Geometry check sheet. Reference: drawing and pictorial views, mm from the part's lowest x, y, z. Give positions to 0.01 mm unless a question says otherwise; leave off trailing zeros. Order: outer loops, then holes, each group sorted by start corner. A loop starts at its lowest first (then second) coordinate and runs counter-clockwise, first axis right, second up.
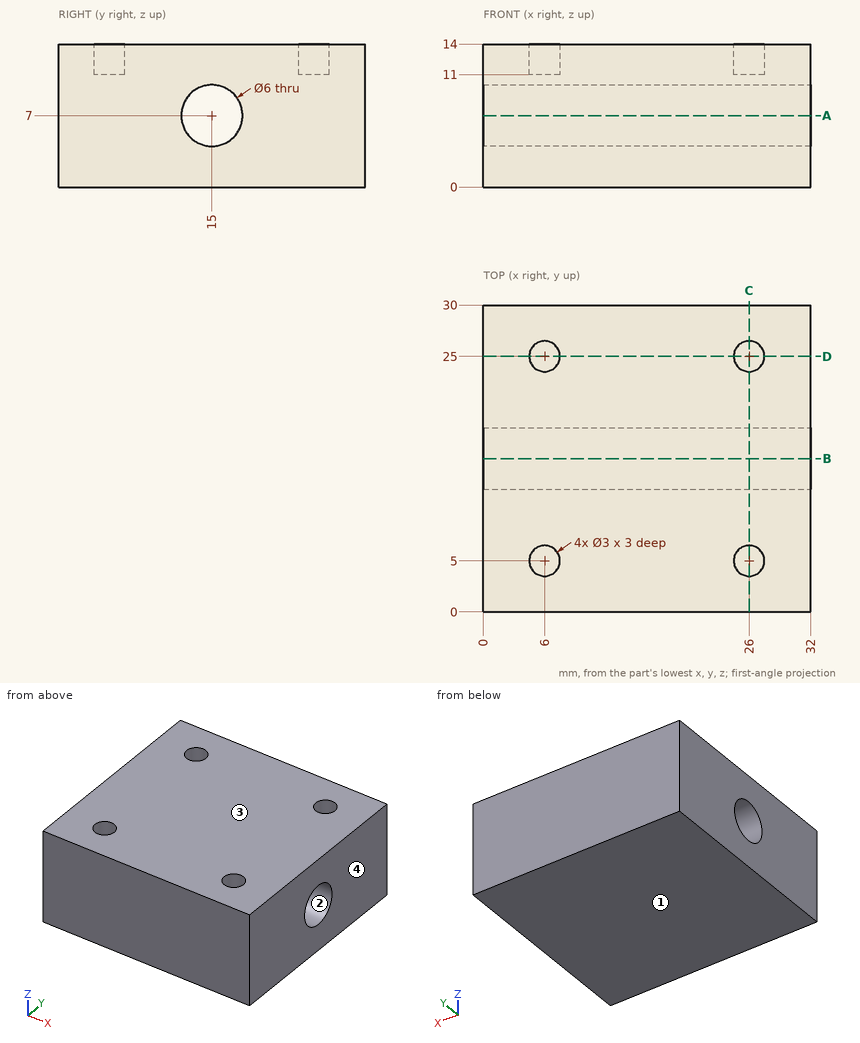
1) Draft check along Z on the marked faces 1, 2, 3 and 4. Enter one of: +Z half, -Z half, draft (parallel to the pull), parting line (faces both ways), or undercut.
Recorded:
face 1: -Z half
face 2: undercut
face 3: +Z half
face 4: draft
2) Section check D-D, the plane y = 25. Record the cut outline in (x, z), then the cut area to 3 significant figures.
Recorded:
outline: (0, 0) - (32, 0) - (32, 14) - (27.5, 14) - (27.5, 11) - (24.5, 11) - (24.5, 14) - (7.5, 14) - (7.5, 11) - (4.5, 11) - (4.5, 14) - (0, 14) - close
area: 430 mm2
3) Depth check by flat-ended pin: pin 1 Ø0.9 at (x, y) = (6, 5) entering from +Z; pin 2 Ø5 at (x, y) = (26, 5) entering from +Z. Enter the tip coordinate at first touch or a pass-through.
Recorded:
pin 1: stops at z = 11
pin 2: stops at z = 14
4) Section check A-A, the plane z = 7. Record the cut outline in (x, y), then the cut area to 3 significant figures.
Recorded:
outline: (0, 0) - (32, 0) - (32, 12) - (0, 12) - close; (0, 18) - (32, 18) - (32, 30) - (0, 30) - close
area: 768 mm2
5) Section check C-C, the plane x = 26. Record the cut outline in (y, z).
Recorded:
outline: (0, 0) - (30, 0) - (30, 14) - (26.5, 14) - (26.5, 11) - (23.5, 11) - (23.5, 14) - (6.5, 14) - (6.5, 11) - (3.5, 11) - (3.5, 14) - (0, 14) - close; hole circle Ø6 at (15, 7)
6) Material ranges on L1, parallel to Y at x = 26, z = 12.15; L2, parallel to X at y = 4.5, z = 13; L3, parallel to Y at x = 21, z = 5, recorded low to high.
Recorded:
L1: y = 0 to 3.5, 6.5 to 23.5, 26.5 to 30
L2: x = 0 to 4.59, 7.41 to 24.59, 27.41 to 32
L3: y = 0 to 12.76, 17.24 to 30
7) Section check B-B, the plane y = 15. Record the cut outline in (x, z).
Recorded:
outline: (0, 0) - (32, 0) - (32, 4) - (0, 4) - close; (0, 10) - (32, 10) - (32, 14) - (0, 14) - close
